Autodesk Inventor part; units mm, degrees
ref_plane "YZ Plane" through (0, 0, 0) normal (1, 0, 0) x (0, 1, 0)
ref_plane "XZ Plane" through (0, 0, 0) normal (0, 1, 0) x (-1, 0, 0)
ref_plane "XY Plane" through (0, 0, 0) normal (0, 0, 1) x (1, 0, 0)
sketch "Sketch1" plane through (0, 0, 0) normal (0, 0, 1) x (1, 0, 0)
  arc A0 (0, 550) -> (-550, 0) centre (0, 0) ccw
  arc A1 (0, 450) -> (-450, 0) centre (0, 0) ccw
  line L0 (0, 550) -> (0, 450)
  line L1 (-450, 0) -> (-550, 0)
  point P0 (-500, 0)
  point P1 (0, 500)
  dimension "d0" = 1100
  dimension "d1" = 900
extrude "Plate1" add sketch "Sketch1" against normal blind 3
sketch "Sketch2" plane through (0, 0, 0) normal (0, 0, 1) x (1, 0, 0)
  line L0 (-550, 0) -> (-450, 0)
  arc A0 (0, 550) -> (-550, 0) centre (0, 0) ccw construction
  circle A1 centre (-480.4174, 198.9954) radius 7
  arc A2 (0, 450) -> (-450, 0) centre (0, 0) ccw construction
  circle A3 centre (0, 0) radius 520 construction
  line L1 (-480.4174, 198.9954) -> (0, 0) construction
  dimension "d17" = 1040
  dimension "d4" = 14
  dimension "d16" = 22.5
extrude "Cut1" cut sketch "Sketch2" against normal through all
pattern_circular "Circular Pattern1" count 2 over 45 about axis through (0, 0, 0) along (0, 0, -1) of "Cut1"
sketch "Sketch3" plane through (0, 0, 0) normal (0, 0, 1) x (1, 0, 0)
  line L0 (-388.9087, 388.9087) -> (-318.1981, 318.1981) construction
  arc A0 (0, 450) -> (-450, 0) centre (0, 0) ccw
  arc A1 (0, 550) -> (-550, 0) centre (0, 0) ccw
  line L1 (-550, 0) -> (-450, 0)
  line L2 (-384.6661, 393.1514) -> (-393.1514, 384.6661)
  line L3 (-384.6661, 393.1514) -> (-349.3107, 357.796)
  line L4 (-393.1514, 384.6661) -> (-357.796, 349.3107)
  line L5 (-357.796, 349.3107) -> (-349.3107, 357.796)
  point P0 (-388.9087, 388.9087)
  dimension "d11" = 45
  dimension "d12" = 12
  dimension "d13" = 50
extrude "Extrusion1" cut sketch "Sketch3" against normal through all
chamfer "Corner Chamfer1" distance 10 angle 45 2 edges at (-384.6429, 393.1282, -1.5) (-393.1282, 384.6429, -1.5)
equation "\"d0\" = Диаметр_вн"
equation "\"d1\" = d0 - 2 * Ширина_кольца"
equation "\"d4\" = Диаметр_отв"
equation "\"d6\" = Thickness"
equation "\"d2\" = Thickness"
equation "\"BendReliefWidth\" = Thickness"
equation "\"BendReliefDepth\" = 0.5 * Thickness"
equation "\"CornerReliefSize\" = 4 * Thickness"
equation "\"MinimumRemnant\" = 2 * Thickness"
equation "\"TransitionRadius\" = BendRadius"
equation "\"JacobiRadiusSize\" = BendRadius"
equation "\"GapSize\" = Thickness"
properties part number "BSH 502 segment" material "Stainless Steel"
Could you check a few things on this model? Use its own coordinates, in mm. A direction names the side the tool comes from. Give positions to 0.01 mm unless a question says otherwise; leave off trailing zeros. Order: outer loops, then holes, each group sorted by start corner. A loop starts at its lowest first (then second) coordinate and runs counter-clockwise, first axis right, second up.
1. Suppose I cut it at A-A (z = -1.6). List the corners of the cut face in (x, y) for me.
2. Suppose I cut it at C-C (x = -295). List the corners of the cut face in (y, z) for me, plus the area to 3 significant figures.
3. For faces 5 (the flat face through (-337, 317, 0)), 6 (the flat face through (-363.639, 372.124, -1.479)), which set-ups out of +Z, -Z, +X, -X, +Y, -Y let a thin tool reach every point of the face, with its end or its side?
4. I need wall thicknesses on L1, parallel to X at y = 483, z = -1; L2, parallel to X at y = 475.5, z = -0.85; L3, parallel to X at y = 266, z = -0.5. Which ranges of each line are inside material? Lowest first, please.
5. Will these pins go through, and if not, where does the flat tip stop? P1, Ø2, axis at x = -206, y = 443, coming from the +Z side; P2, Ø1.5, axis at x = -242, z = -2.5, coming from the -Y side.
6. We'd pull the mould along X, two halves only. Please class faces 1 (the cylindrical face through (-200.35, 512.21, -1.48)), 2 (the cylindrical face through (-481.93, 192.16, -1.48)), 3 (the cylindrical face through (-314.68, 321.68, -1.48)), 4 (the flat face through (-337, 317, -3)): pulls with the +X half, pulls with the -X half, needs draft (parallel to the pull), parting line crosses it, or undercut.
7. Suppose I cut it at B-B (y = 68). List the corners of the cut face in (x, z) for me.
Solved:
1. outline: (-550, 0) - (-450, 0) arc R450 cw to (0, 450) - (0, 550) arc R550 ccw to (-377.43, 400.06) - (-377.57, 386.06) - (-349.31, 357.8) - (-357.8, 349.31) - (-386.06, 377.57) - (-400.06, 377.43) arc R550 ccw to start; hole circle Ø14 at (-480.42, 199); hole circle Ø14 at (-199, 480.42)
2. outline: (339.82, -3) - (464.19, -3) - (464.19, 0) - (339.82, 0) - close
2. area: 373 mm2
3. face 5: +Z, +X, -X, +Y, -Y
3. face 6: +Z, -Z
4. L1: x = -263.08 to -205.5, -192.49 to 0
4. L2: x = -276.41 to -203.98, -194.01 to 0
4. L3: x = -481.4 to -362.97
5. P1: stops at z = 0
5. P2: stops at y = 378.91
6. face 1: pulls with the -X half
6. face 2: undercut
6. face 3: pulls with the +X half
6. face 4: needs draft
7. outline: (-545.78, -3) - (-444.83, -3) - (-444.83, 0) - (-545.78, 0) - close
